The model under review builds one solid part; all positions refer to its coordinate system, in mm. Face numbers are marked on the shaded views. A direction names the side the tool comes from. Coordinates: 2 decimals unless noted, no trailing zeros. Order: outer loops, then holes, each group sorted by start corner. A loop starts at its lowest first (then second) coordinate and runs counter-clockwise, first axis right, second up. Notation, with made-up numbers: M 41.5,27.25 L 91.5,27.25 A22 ccw 91.5,51.25 Z; hole C -32,29.25 d1. An arc over 180 degrees is marked long. Write each question's results on one line, items separated by ' | '.
from build123d import *

# Parameters (mm, degrees)
SKETCH1_W           = 18.5
SKETCH1_H           = 10
BOSS_EXTRUDE1_DEPTH = 10
SKETCH2_W           = 10
SKETCH2_H           = 10
BOSS_EXTRUDE2_DEPTH = 50
SKETCH3_W           = 18.5
SKETCH3_H           = 10
BOSS_EXTRUDE3_DEPTH = 10
SKETCH4_R           = 1.75
CUT_EXTRUDE1_DEPTH  = 71.785326869
SKETCH5_R           = 1.75
CUT_EXTRUDE2_DEPTH  = 72.313129927


with BuildPart() as part:
    # Sketch1 → Boss-Extrude1 (new body)
    with BuildSketch(Plane.XY):
        Rectangle(SKETCH1_W, SKETCH1_H)
    extrude(amount=BOSS_EXTRUDE1_DEPTH)

    # Sketch2 → Boss-Extrude2 (add)
    with BuildSketch(Plane.XY.offset(10)):
        with Locations((-4.25, 0)):
            Rectangle(SKETCH2_W, SKETCH2_H)
    extrude(amount=BOSS_EXTRUDE2_DEPTH)

    # Sketch3 → Boss-Extrude3 (add)
    with BuildSketch(Plane.XY.offset(60)):
        Rectangle(SKETCH3_W, SKETCH3_H)
    extrude(amount=BOSS_EXTRUDE3_DEPTH)

    # Sketch4 → Cut-Extrude1 (cut, through all)
    with BuildSketch(Plane.XY.offset(70)):
        with Locations((5.25, 0)):
            Circle(SKETCH4_R)
    extrude(amount=-CUT_EXTRUDE1_DEPTH, mode=Mode.SUBTRACT)

    # Sketch5 → Cut-Extrude2 (cut, through all)
    with BuildSketch(Plane(origin=(0, 5, 0), x_dir=(1, 0, 0), z_dir=(0, 1, 0))):
        with Locations(Location((-4.25, -23, 0), (0, 0, 270))):
            Circle(SKETCH5_R)
        with Locations(Location((-4.25, -47, 0), (0, 0, 270))):
            Circle(SKETCH5_R)
    extrude(amount=-CUT_EXTRUDE2_DEPTH, mode=Mode.SUBTRACT)


solid = part.part
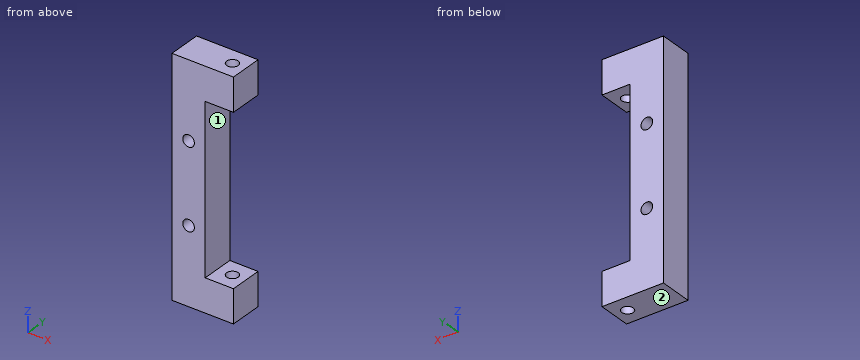
1) Take a section at C-C on x = -4.25. State the section outline as (y, z) points, plus the area to 3 significant figures.
Solutions:
outline: M -5,0 L 5,0 L 5,21.25 L -5,21.25 Z; M -5,24.75 L 5,24.75 L 5,45.25 L -5,45.25 Z; M -5,48.75 L 5,48.75 L 5,70 L -5,70 Z | area: 630 mm2
2) Take a section at A-A on y = 0. State the section outline as (x, z) points, plus the area to 3 significant figures.
Solutions:
outline: M -9.25,0 L 3.5,0 L 3.5,10 L 0.75,10 L 0.75,60 L 3.5,60 L 3.5,70 L -9.25,70 Z; M 7,0 L 9.25,0 L 9.25,10 L 7,10 Z; M 7,60 L 9.25,60 L 9.25,70 L 7,70 Z; hole C -4.25,23 d3.5; hole C -4.25,47 d3.5 | area: 781 mm2
3) Take a section at B-B on z = 23. State the section outline as (x, y) points.
Solutions:
outline: M -9.25,-5 L -6,-5 L -6,5 L -9.25,5 Z; M -2.5,-5 L 0.75,-5 L 0.75,5 L -2.5,5 Z
4) For the marked faces 1 and 2, list the 3-axis set-ups (+Z, -Z, +X, -X, +Y, -Y) from which the entire face can be reached by the end or side of a thin tool; tool diameter is ignored.
Solutions:
face 1: +X, +Y, -Y | face 2: -Z, +X, -X, +Y, -Y
5) Take a section at D-D on y = 3. State the section outline as (x, z) points, plus the area to 3 significant figures.
Solutions:
outline: M -9.25,0 L 9.25,0 L 9.25,10 L 0.75,10 L 0.75,60 L 9.25,60 L 9.25,70 L -9.25,70 Z; hole C -4.25,23 d3.5; hole C -4.25,47 d3.5 | area: 851 mm2
6) For pin 1 (3 mm diameter, centred on y = -1, z = 43, fed in from +X), flat-tipped, find the tip position at first contact; note if it passes through.
Solutions:
pin 1: x = 0.75
7) To check wall thickness, follow line 1 along Z through (x, y) = (2.5, 1.25); line 2 along Z through (x, y) = (-4.75, 3.5); line 3 along Y through (x, z) = (5.25, 66). State the ranges of each line that lie inside material, in increasing order.
Solutions:
line 1: 0 to 10, 60 to 70 | line 2: 0 to 21.32, 24.68 to 45.32, 48.68 to 70 | line 3: -5 to -1.75, 1.75 to 5
